For this review, take the finished solid that the model builds, in its own axes (mm). A direction names the side the tool comes from. Round coordinates to 2 decimals unless told otherwise and drop trailing zeros. Write each loop counter-clockwise with the first axis right and the second up, starting at its lowest first coordinate (ties: lowest second). Pieces come first, ordered by that corner, then holes. Notation, with made-up numbers: M 24,72 L 60,72 A25 cw 60,94 Z; hole C 13,47 d7. An arc over 180 degrees is marked long. One line per question, with ' | ' between items.
```python
from build123d import *

# Parameters (mm, degrees)
SKETCH_1_R          = 10
EXTRUDE_1_DEPTH     = 12.5
SKETCH_2_R          = 4
CUT_EXTRUDE_1_DEPTH = 12.5
SKETCH_4_W          = 53.049184892
SKETCH_4_H          = 1
CUT_EXTRUDE_2_DEPTH = 25
SKETCH_5_W          = 15.903552991
SKETCH_5_H          = 1
CUT_EXTRUDE_3_DEPTH = 25
SKETCH_6_R          = 2.5
CUT_EXTRUDE_4_DEPTH = 25


with BuildPart() as part:
    # 草图1 → 凸台-拉伸1 (new body, symmetric)
    with BuildSketch(Plane.XY):
        Circle(SKETCH_1_R)
    extrude(amount=EXTRUDE_1_DEPTH, both=True)

    # 草图2 → 切除-拉伸1 (cut)
    with BuildSketch(Plane.XY.offset(12.5)):
        Circle(SKETCH_2_R)
    extrude(amount=-CUT_EXTRUDE_1_DEPTH, mode=Mode.SUBTRACT)

    # 草图4 → 切除-拉伸2 (cut)
    with BuildSketch(Plane(origin=(0, 0, 0), x_dir=(1, 0, 0), z_dir=(0, 1, 0))):
        Rectangle(SKETCH_4_W, SKETCH_4_H)
    extrude(amount=-CUT_EXTRUDE_2_DEPTH, mode=Mode.SUBTRACT)

    # 草图5 → 切除-拉伸3 (cut)
    with BuildSketch(Plane.XY.offset(12.5)):
        with Locations((-7.951776496, -0.5)):
            Rectangle(SKETCH_5_W, SKETCH_5_H)
    extrude(amount=-CUT_EXTRUDE_3_DEPTH, mode=Mode.SUBTRACT)

    # 草图6 → 切除-拉伸4 (cut)
    with BuildSketch(Plane(origin=(0, 0, -12.5), x_dir=(-1, 0, 0), z_dir=(0, 0, -1))):
        Circle(SKETCH_6_R)
    extrude(amount=-CUT_EXTRUDE_4_DEPTH, mode=Mode.SUBTRACT)


solid = part.part
```
Item 1: Take a section at B-B (x = 0). Write out the cut boundary in (y, z).
Results:
outline: M -10,-12.5 L -2.5,-12.5 L -2.5,-0.5 L -10,-0.5 Z; M -10,0.5 L -4,0.5 L -4,12.5 L -10,12.5 Z; M 2.5,-12.5 L 10,-12.5 L 10,12.5 L 4,12.5 L 4,0 L 2.5,0 Z
Item 2: Insertion check: pin 1 Ø3 at (y, z) = (-5, 3) entering from -X; pin 2 Ø2 at (x, z) = (-5, 2.5) entering from -Y; pin 3 Ø6 at (y, z) = (-4.5, -2.5) entering from -X; pin 4 Ø6 at (x, y) = (1.5, 0.5) entering from -Z. Each pin has a flat end and moves straight along its axis. Give the tip position at first contact, or say it passes through.
Results:
pin 1: x = -9.37 | pin 2: y = -9.17 | pin 3: x = -9.89 | pin 4: z = -12.5
Item 3: Take a section at C-C (y = -3.25). Write out the cut boundary in (x, z), then the cut area to 3 significant figures.
Results:
outline: M -9.46,-12.5 L 9.46,-12.5 L 9.46,-0.5 L -9.46,-0.5 Z; M -9.46,0.5 L -2.33,0.5 L -2.33,12.5 L -9.46,12.5 Z; M 2.33,0.5 L 9.46,0.5 L 9.46,12.5 L 2.33,12.5 Z | area: 398 mm2
Item 4: To check wall thickness, follow line 1 along Y through (x, z) = (0, -4.25); line 2 along Z through (x, y) = (3.5, -7); line 3 along X through (y, z) = (-1.25, 7.25). State the ranges of each line that lie inside material, in increasing order. Write a range as from..to.
Results:
line 1: -10..-2.5, 2.5..10 | line 2: -12.5..-0.5, 0.5..12.5 | line 3: -9.92..-3.8, 3.8..9.92
Item 5: Mouldability with a two-part tool opening along X and no side actions: class faces 4 (the face through (0, -5, -0.5)), 5 (the face through (8, 6, 0)), 6 (the face through (0, 3, 0)) as +X half, -X half, draft (parallel to the pull), parting line (faces both ways), or undercut.
Results:
face 4: draft | face 5: parting line | face 6: undercut
Item 6: Take a section at A-A (y = -8). Write out the cut boundary in (x, z), then the cut area to 3 significant figures.
Results:
outline: M -6,-12.5 L 6,-12.5 L 6,-0.5 L -6,-0.5 Z; M -6,0.5 L 6,0.5 L 6,12.5 L -6,12.5 Z | area: 288 mm2
Item 7: Take a section at D-D (x = 7). Write out the cut boundary in (y, z).
Results:
outline: M -7.14,-12.5 L 7.14,-12.5 L 7.14,12.5 L -7.14,12.5 L -7.14,0.5 L 0,0.5 L 0,-0.5 L -7.14,-0.5 Z
Item 8: Machinability: for faces 1 (the face through (-6, 0, 0)), 2 (the face through (-0.1, -4.3, 12.5)), 3 (the face through (6, 0, 0)), which of the approach directions +Z, -Z, +X, -X, +Y, -Y give a long, thin tool a straight path to every point of the face, cutting with its end or side? Answer none if there is none.
Results:
face 1: +Z, -Z, -X | face 2: +Z, +X, -X, +Y, -Y | face 3: +X, -X, -Y
